Verification items for the finished model (mm, model axes). Face numbers are marked on the shaded views. A direction names the side the tool comes from. Give positions to 0.01 mm unless a question says otherwise; leave off trailing zeros. Order: outer loops, then holes, each group sorted by start corner. A loop starts at its lowest first (then second) coordinate and runs counter-clockwise, first axis right, second up. Notation, with made-up numbers: (62, 30.5) -> (83, 30.5) arc R34 ccw to (83, 69.5) -> close; hole circle Ø2 at (23, 39.25). An arc over 180 degrees is marked (long way). Return JSON: item names as keys, results as strings. Group by question number.
(1) Cross-section at D-D on y = 1.5. Enter the section's corners in (x, z), then the cut area to 3 significant figures.
(2) Thickness scan on line 1 along Z through (x, y) = (18.75, -1.5); line 2 along Y through (x, z) = (0, 15); line 3 along X through (y, z) = (6.75, 8.75). Record the ranges inside material, lowest first.
(3) Release check for a two-part mould opening along Y. For the marked faces 1, 2, 3 and 4 record: pulls with the +Y half, pulls with the -Y half, needs draft (parallel to the pull), parting line crosses it, or undercut.
(4) Cross-section at A-A on z = 15. Enter the section's corners in (x, y), then the cut area to 3 significant figures.
(5) Tool access check on the marked faces 5 and 6. Record the directions out of +Z, -Z, +X, -X, +Y, -Y that give a thin tool (end or side, any length) a straight path to the whole face; none if there is none.
(6) Cross-section at B-B on x = 18.75. Enter the section's corners in (y, z), then the cut area to 3 significant figures.
(7) Cross-section at C-C on z = 26.25. Enter the section's corners in (x, y).
(8) Depth check by flat-ended pin: pin 1 Ø4 at (x, z) = (-19.5, 12) entering from +Y; pin 2 Ø8.5 at (y, z) = (11, 21) entering from -X; pin 3 Ø3 at (y, z) = (13.5, 16) entering from +X. Enter the tip coordinate at first touch or a pass-through.
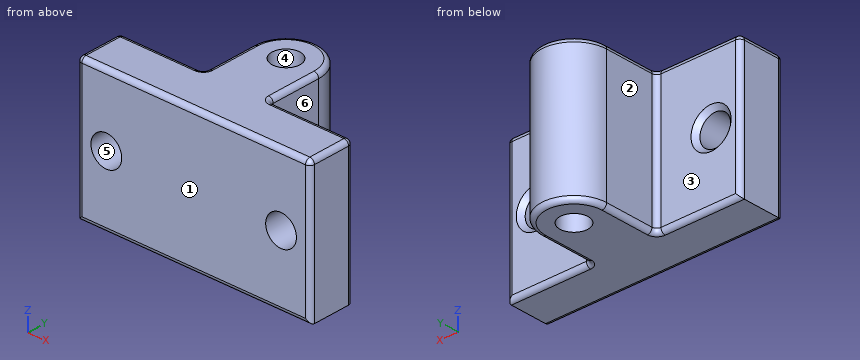
from build123d import *

# Parameters (mm, degrees)
SKETCH1_W           = 50
SKETCH1_H           = 10
BOSS_EXTRUDE1_DEPTH = 30
SKETCH2_R           = 3
BOSS_EXTRUDE2_DEPTH = 30
CUT_EXTRUDE1_REACH  = 45.277
SKETCH3_R           = 3.3
FILLET1_R           = 1
CHAMFER1_SIZE       = 1


with BuildPart() as part:
    # Sketch1 → Boss-Extrude1 (new body)
    with BuildSketch(Plane.XY):
        Rectangle(SKETCH1_W, SKETCH1_H)
    extrude(amount=BOSS_EXTRUDE1_DEPTH)

    # Sketch2 → Boss-Extrude2 (add)
    with BuildSketch(Plane.XY.offset(30)):
        with BuildLine():
            Line((-7, 5), (-7, 16.65178901))
            ThreePointArc((-7, 16.65178901), (0, 23.65178901), (7, 16.65178901))
            Line((7, 16.65178901), (7, 5))
            Line((7, 5), (-7, 5))
        make_face()
        with Locations((0, 16.65178901)):
            Circle(SKETCH2_R, mode=Mode.SUBTRACT)
    extrude(amount=-BOSS_EXTRUDE2_DEPTH)

    # Sketch3 → Cut-Extrude1 (cut, up to next)
    with BuildSketch(Plane(origin=(0, 5, 0), x_dir=(1, 0, 0), z_dir=(0, 1, 0)), mode=Mode.PRIVATE) as cut_extrude1_sk1:
        with Locations(Location((-18.75, -15, 0), (0, 0, 180))):
            Circle(SKETCH3_R)
    cut_extrude1_tool1 = extrude(cut_extrude1_sk1.sketch, amount=-CUT_EXTRUDE1_REACH, mode=Mode.PRIVATE) & part.part
    # Sketch3 → Cut-Extrude1 (cut, up to next)
    with BuildSketch(Plane(origin=(0, 5, 0), x_dir=(1, 0, 0), z_dir=(0, 1, 0)), mode=Mode.PRIVATE) as cut_extrude1_sk2:
        with Locations(Location((18.75, -15, 0), (0, 0, 180))):
            Circle(SKETCH3_R)
    cut_extrude1_tool2 = extrude(cut_extrude1_sk2.sketch, amount=-CUT_EXTRUDE1_REACH, mode=Mode.PRIVATE) & part.part
    add(cut_extrude1_tool1.solids().sort_by_distance((-18.75, 5, 15))[0], mode=Mode.SUBTRACT)
    add(cut_extrude1_tool2.solids().sort_by_distance((18.75, 5, 15))[0], mode=Mode.SUBTRACT)

    # Fillet1
    fillet1_edges = [part.edges().sort_by_distance(p)[0] for p in [
        (25, 0, 30),
        (-16, 5, 0),
        (-16, 5, 30),
        (16, 5, 30),
        (-7, 5, 15),
        (7, 5, 15),
        (7, 10.825894505, 30),
        (0, 23.65178901, 30),
        (-7, 10.825894505, 30),
        (-7, 10.825894505, 0),
        (0, 23.65178901, 0),
        (7, 10.825894505, 0),
        (-25, 0, 30),
        (16, 5, 0),
        (0, -5, 0),
        (-25, 5, 15),
        (25, 5, 15),
        (25, -5, 15),
        (-25, -5, 15),
        (0, -5, 30),
    ]]
    fillet(fillet1_edges, radius=FILLET1_R)

    # Chamfer1
    chamfer1_edges = [part.edges().sort_by_distance(p)[0] for p in [
        (-15.45, 5, 15),
        (22.05, 5, 15),
    ]]
    chamfer(chamfer1_edges, length=CHAMFER1_SIZE)


solid = part.part
Verdict:
{
 "1": {"outline": "(-25, 0) -> (25, 0) -> (25, 29) arc R1 ccw to (24, 30) -> (-24, 30) arc R1 ccw to (-25, 29) -> close; hole circle Ø6.6 at (-18.75, 15); hole circle Ø6.6 at (18.75, 15)", "area": "1,430 mm²"},
 "2": {"line 1": "0 to 11.7, 18.3 to 30", "line 2": "-5 to 13.65, 19.65 to 23.65", "line 3": "-7 to 7"},
 "3": {"face 1": "pulls with the -Y half", "face 2": "needs draft", "face 3": "pulls with the +Y half", "face 4": "undercut"},
 "4": {"outline": "(-25, -4) arc R1 ccw to (-24, -5) -> (-22.05, -5) -> (-22.05, 4) -> (-23.05, 5) -> (-24, 5) arc R1 ccw to (-25, 4) -> close; (-15.45, -5) -> (15.45, -5) -> (15.45, 4) -> (14.45, 5) -> (8, 5) arc R1 cw to (7, 6) -> (7, 16.65) arc R7 ccw to (-7, 16.65) -> (-7, 6) arc R1 cw to (-8, 5) -> (-14.45, 5) -> (-15.45, 4) -> close; (22.05, -5) -> (24, -5) arc R1 ccw to (25, -4) -> (25, 4) arc R1 ccw to (24, 5) -> (23.05, 5) -> (22.05, 4) -> close; hole circle Ø6 at (0, 16.65)", "area": "577 mm²"},
 "5": {"face 5": "+Y, -Y", "face 6": "+Z, -Z, +X, +Y"},
 "6": {"outline": "(-5, 1) arc R1 ccw to (-4, 0) -> (4, 0) arc R1 ccw to (5, 1) -> (5, 10.7) -> (4, 11.7) -> (-5, 11.7) -> close; (-5, 18.3) -> (4, 18.3) -> (5, 19.3) -> (5, 29) arc R1 ccw to (4, 30) -> (-4, 30) arc R1 ccw to (-5, 29) -> close", "area": "232 mm²"},
 "7": {"outline": "(-25, -4) arc R1 ccw to (-24, -5) -> (24, -5) arc R1 ccw to (25, -4) -> (25, 4) arc R1 ccw to (24, 5) -> (8, 5) arc R1 cw to (7, 6) -> (7, 16.65) arc R7 ccw to (-7, 16.65) -> (-7, 6) arc R1 cw to (-8, 5) -> (-24, 5) arc R1 ccw to (-25, 4) -> close; hole circle Ø6 at (0, 16.65)"},
 "8": {"pin 1": "y = 5", "pin 2": "x = -7", "pin 3": "x = 7"}
}
